The model under review builds one solid part; all positions refer to its coordinate system, in mm. A direction names the side the tool comes from. Give positions to 0.01 mm unless a question says otherwise; leave off trailing zeros. Order: outer loops, then holes, each group sorted by start corner. A loop starts at its lowest first (then second) coordinate and runs counter-clockwise, first axis right, second up. Notation, with made-up numbers: (-20, 5) - (-15, 5) arc R23 ccw to (-15, 42) - close; hole circle Ø4 at (87.5, -36). An arc over 180 degrees is marked (long way). Use CSV: the item, a comma, the result in double quotes. Start each with the question number.
1. Take a section at A-A, the plane x = 0. State the section outline as (y, z) points, then the cut area to 3 significant figures.
2. Take a section at C-C, the plane y = 5.5. State the section outline as (x, z) points.
3. For pin 1 (1.5 mm diameter, centred on y = 1, z = 5, fed in from -X); pin 2 (1.5 mm diameter, centred on x = 4.5, z = 21.5, fed in from +Y); pin 3 (1 mm diameter, centred on x = -4, z = 10, fed in from +Y), all flat-tipped, find the tip position at first contact; note any pin that passes through.
4. To check wall thickness, follow line 1 (Y direction, x = 0, z = 13.25); line 2 (Z direction, x = -5.25, y = -1.25); line 3 (X direction, y = -1.75, z = 3.25). State the ranges of each line that lie inside material, in increasing order. Write a range as [from, to].
5. Draft analysis for pull direction Y (two halves, no side actions). For faces 4 (the flat face through (6.12, 3.91, 7.96)), 5 (the flat face through (-7.24, -0.01, 7.96)), 6 (the cylindrical face through (-0.01, -6.35, 7.74)), state which applies: released by +Y, released by -Y, zero draft, split by the parting line, or undercut.
6. Machinability: for faces 1 (the cylindrical face through (-1.782, 6.095, 7.74)), 2 (the flat face through (-1.05, -7.18, 7.96)), 3 (the cylindrical face through (6.286, 0.896, 7.74)), which of the approach directions +Z, -Z, +X, -X, +Y, -Y give a long, thin tool a straight path to every point of the face, cutting with its end or side? Answer none if there is none.
7. Take a section at B-B, the plane y = 0. State the section outline as (x, z) points.
```python
from build123d import *

# Parameters (mm, degrees)
SKETCH1_R           = 6.35
BOSS_EXTRUDE1_DEPTH = 15.7
BOSS_EXTRUDE2_DEPTH = 15.7
CIRPATTERN1_COUNT   = 11
SKETCH3_R           = 5.08
BOSS_EXTRUDE3_DEPTH = 8.62
SKETCH4_R           = 2.5
CUT_EXTRUDE1_DEPTH  = 25.32


with BuildPart() as part:
    # Sketch1 → Boss-Extrude1 (new body)
    with BuildSketch(Plane.XY):
        Circle(SKETCH1_R)
    extrude(amount=BOSS_EXTRUDE1_DEPTH)

    # Sketch2 → Boss-Extrude2 (add)
    with BuildSketch(Plane.XY.offset(15.7)):
        Polygon((0, 8.13319935), (-0.762, 8.13319935), (-1.388433627, 5.795317226), (1.388433627, 5.795317226), (0.762, 8.13319935), align=None)
    boss_extrude2 = extrude(amount=-BOSS_EXTRUDE2_DEPTH)

    # CirPattern1: Boss-Extrude2 ×11 about axis
    cirpattern1_axis = Axis((0, 0, 0), (0, 0, 1))
    for i in range(1, CIRPATTERN1_COUNT):
        add(boss_extrude2.rotate(cirpattern1_axis, i * 360 / CIRPATTERN1_COUNT))

    # Sketch3 → Boss-Extrude3 (add)
    with BuildSketch(Plane.XY.offset(15.7)):
        Circle(SKETCH3_R)
    extrude(amount=BOSS_EXTRUDE3_DEPTH)

    # Sketch4 → Cut-Extrude1 (cut, through all)
    with BuildSketch(Plane.XY.offset(24.32)):
        Circle(SKETCH4_R)
    extrude(amount=-CUT_EXTRUDE1_DEPTH, mode=Mode.SUBTRACT)


solid = part.part
```
Determined:
1,outline,"(-6.35, 0) - (-2.5, 0) - (-2.5, 24.32) - (-5.08, 24.32) - (-5.08, 15.7) - (-6.35, 15.7) - close; (2.5, 0) - (8.13, 0) - (8.13, 15.7) - (5.08, 15.7) - (5.08, 24.32) - (2.5, 24.32) - close"
1,area,"193 mm²"
2,outline,"(-4.74, 0) - (4.74, 0) - (4.74, 15.7) - (-4.74, 15.7) - close"
3,pin 1,"stops at x = -6.63"
3,pin 2,"stops at y = 3.43"
3,pin 3,"stops at y = 7.25"
4,line 1,"y = [-6.35, -2.5], [2.5, 8.13]"
4,line 2,"z = [0, 15.7]"
4,line 3,"x = [-7.97, -1.79], [1.79, 7.97]"
5,face 4,"released by +Y"
5,face 5,"undercut"
5,face 6,"released by -Y"
6,face 1,"+Z, -Z, +Y"
6,face 2,"+Z, -Z, -Y"
6,face 3,"+Z, -Z, +X"
7,outline,"(-7.22, 0) - (-2.5, 0) - (-2.5, 24.32) - (-5.08, 24.32) - (-5.08, 15.7) - (-7.22, 15.7) - close; (2.5, 0) - (7.22, 0) - (7.22, 15.7) - (5.08, 15.7) - (5.08, 24.32) - (2.5, 24.32) - close"
